Check sheet for the modelled part. Datum: model origin and axes. Units: mm. A direction names the side the tool comes from. Coordinates: 2 decimals unless noted, no trailing zeros. Order: outer loops, then holes, each group sorted by start corner. A loop starts at its lowest first (then second) coordinate and runs counter-clockwise, first axis right, second up.
from build123d import *

# Parameters (mm, degrees)
F1_DEPTH = 120
F3_D     = 2.7
F3_DEPTH = 12
F3_TIP   = 0.8111618357
F4_W     = 9
F4_H     = 9
F5_DEPTH = 5
F7_D     = 2.7
F7_DEPTH = 5
F7_TIP   = 0.8111618357
F9_DEPTH = 50


with BuildPart() as f1:
    # F0 (on Front) → F1 (new body)
    with BuildSketch(Plane.XZ):
        with BuildLine():
            Line((-10.0352883258, -17.0069661875), (0, -17.0069661875))
            Line((0, -17.0069661875), (10.0352883258, -17.0069661875))
            Line((10.0352883258, -17.0069661875), (7, -12.5069661875))
            Line((7, -12.5069661875), (46.25, -12.5069661875))
            Line((46.25, -12.5069661875), (43.2147116742, -17.0069661875))
            Line((43.2147116742, -17.0069661875), (53.2852883258, -17.0069661875))
            Line((53.2852883258, -17.0069661875), (50.25, -12.5069661875))
            Line((50.25, -12.5069661875), (55.25, -12.5069661875))
            ThreePointArc((55.25, -12.5069661875), (57.3713203436, -11.6282865311), (58.25, -9.5069661875))
            Line((58.25, -9.5069661875), (58.25, 21.9930338125))
            ThreePointArc((58.25, 21.9930338125), (57.3713203436, 24.114354156), (55.25, 24.9930338125))
            Line((55.25, 24.9930338125), (50.8726710718, 24.9930338125))
            Line((50.8726710718, 24.9930338125), (53.5, 20.9930338125))
            Line((53.5, 20.9930338125), (48.25, 20.9930338125))
            Line((48.25, 20.9930338125), (48.25, 1.6930338125))
            Line((48.25, 1.6930338125), (51.1, 1.6930338125))
            Line((51.1, 1.6930338125), (51.1, -0.5069661875))
            Line((51.1, -0.5069661875), (48.25, -0.5069661875))
            Line((48.25, -0.5069661875), (48.25, -3.5069661875))
            ThreePointArc((48.25, -3.5069661875), (47.3713203436, -5.6282865311), (45.25, -6.5069661875))
            Line((45.25, -6.5069661875), (0, -6.5069661875))
            Line((0, -6.5069661875), (-45.25, -6.5069661875))
            ThreePointArc((-45.25, -6.5069661875), (-47.3713203436, -5.6282865311), (-48.25, -3.5069661875))
            Line((-48.25, -3.5069661875), (-48.25, -0.5069661875))
            Line((-48.25, -0.5069661875), (-51.1, -0.5069661875))
            Line((-51.1, -0.5069661875), (-51.1, 1.6930338125))
            Line((-51.1, 1.6930338125), (-48.25, 1.6930338125))
            Line((-48.25, 1.6930338125), (-48.25, 20.9930338125))
            Line((-48.25, 20.9930338125), (-53.5, 20.9930338125))
            Line((-53.5, 20.9930338125), (-50.8726710718, 24.9930338125))
            Line((-50.8726710718, 24.9930338125), (-55.25, 24.9930338125))
            ThreePointArc((-55.25, 24.9930338125), (-57.3713203436, 24.114354156), (-58.25, 21.9930338125))
            Line((-58.25, 21.9930338125), (-58.25, -9.5069661875))
            ThreePointArc((-58.25, -9.5069661875), (-57.3713203436, -11.6282865311), (-55.25, -12.5069661875))
            Line((-55.25, -12.5069661875), (-50.25, -12.5069661875))
            Line((-50.25, -12.5069661875), (-53.2852883258, -17.0069661875))
            Line((-53.2852883258, -17.0069661875), (-43.2147116742, -17.0069661875))
            Line((-43.2147116742, -17.0069661875), (-46.25, -12.5069661875))
            Line((-46.25, -12.5069661875), (-7, -12.5069661875))
            Line((-7, -12.5069661875), (-10.0352883258, -17.0069661875))
        make_face()
        Polygon((-54, -3.1069661875), (-54, -1.4069661875), (-52.4, -1.4069661875), (-52.4, -3.1069661875), (-50.7, -3.1069661875), (-50.7, -4.7069661875), (-52.4, -4.7069661875), (-52.4, -6.4069661875), (-54, -6.4069661875), (-54, -4.7069661875), (-55.7, -4.7069661875), (-55.7, -3.1069661875), align=None, mode=Mode.SUBTRACT)
        Polygon((52.4, -1.4069661875), (54, -1.4069661875), (54, -3.1069661875), (55.7, -3.1069661875), (55.7, -4.7069661875), (54, -4.7069661875), (54, -6.4069661875), (52.4, -6.4069661875), (52.4, -4.7069661875), (50.7, -4.7069661875), (50.7, -3.1069661875), (52.4, -3.1069661875), align=None, mode=Mode.SUBTRACT)
        Polygon((-55.7, 15.5930338125), (-55.7, 17.1930338125), (-54, 17.1930338125), (-54, 18.8930338125), (-52.4, 18.8930338125), (-52.4, 17.1930338125), (-50.7, 17.1930338125), (-50.7, 15.5930338125), (-52.4, 15.5930338125), (-52.4, 13.8930338125), (-54, 13.8930338125), (-54, 15.5930338125), align=None, mode=Mode.SUBTRACT)
        Polygon((54, 18.8930338125), (54, 17.1930338125), (55.7, 17.1930338125), (55.7, 15.5930338125), (54, 15.5930338125), (54, 13.8930338125), (52.4, 13.8930338125), (52.4, 15.5930338125), (50.7, 15.5930338125), (50.7, 17.1930338125), (52.4, 17.1930338125), (52.4, 18.8930338125), align=None, mode=Mode.SUBTRACT)
    extrude(amount=-F1_DEPTH)

    # F3
    with Locations(Plane.XZ):
        with Locations((0, -15.5069661875)):
            Hole(F3_D / 2, depth=F3_DEPTH)
            with Locations((0, 0, -(F3_DEPTH + F3_TIP / 2))):  # 118° drill point
                Cone(0, F3_D / 2, F3_TIP, mode=Mode.SUBTRACT)

    # F4 (on face) → F5 (join)
    with BuildSketch(Plane.XY.offset(-6.5069661875)):
        with Locations((-10.75, 14.5)):
            Rectangle(F4_W, F4_H)
        with Locations((-10.75, 106.5)):
            Rectangle(F4_W, F4_H)
        with Locations((37.25, 14.5)):
            Rectangle(F4_W, F4_H)
        with Locations((37.25, 106.5)):
            Rectangle(F4_W, F4_H)
    extrude(amount=F5_DEPTH)

    # F7
    with Locations(Plane.XY.offset(-1.5069661875)):
        with Locations((-10.75, 106.5), (37.25, 106.5), (-10.75, 14.5), (37.25, 14.5)):
            Hole(F7_D / 2, depth=F7_DEPTH)
            with Locations((0, 0, -(F7_DEPTH + F7_TIP / 2))):  # 118° drill point
                Cone(0, F7_D / 2, F7_TIP, mode=Mode.SUBTRACT)

    # F8 (on face) → F9 (join)
    with BuildSketch(Plane(origin=(0, 120, 0), x_dir=(-1, 0, 0), z_dir=(0, 1, 0))):
        Polygon((21.25, -1.0069661875), (21.25, -6.5069661875), (25.5, -6.5069661875), (25.5, -4.5069661875), (22.75, -4.5069661875), (22.75, -2.7069661875), (25.5, -2.7069661875), (25.5, -1.0069661875), align=None)
        Polygon((41, -4.5069661875), (41, -6.5069661875), (45.25, -6.5069661875), (45.25, -1.0069661875), (41, -1.0069661875), (41, -2.7069661875), (43.75, -2.7069661875), (43.75, -4.5069661875), align=None)
    extrude(amount=-F9_DEPTH)


solid = f1.part
(1) Release check for a two-part mould opening along Y. For faces 1 (the conical face through (37.47, 14.57, -7.18)), 2 (the cylindrical face through (0.18, 6.08, -14.17)), 3 (the cylindrical face through (-11.37, 105.3, -4.04)) record: +Y half, -Y half, draft (parallel to the pull), parting line (faces both ways), or undercut.
Filled in:
face 1: undercut
face 2: draft
face 3: undercut
(2) Cross-section at A-A (z = 11.5). Enter the section's corners in (x, y).
Filled in:
outline: (-58.25, 0) - (-48.25, 0) - (-48.25, 120) - (-58.25, 120) - close; (48.25, 0) - (58.25, 0) - (58.25, 120) - (48.25, 120) - close
(3) Cross-section at B-B (y = 49). Count the separate pieces of the cut face and the enclosed holes in it, and give its area (3 significant figures).
Filled in:
separate pieces: 1
enclosed holes: 4
area: 1,370 mm2
(4) Cross-section at C-C (x = -4). Enter the section's corners in (y, z).
Filled in:
outline: (0, -17.01) - (120, -17.01) - (120, -6.51) - (0, -6.51) - close
(5) Go/stop test with flat-tipped pins: P1, Ø0.9, axis at x = 54.5, y = 31, coming from the -Z side; P2, Ø10, axis at x = -11.5, y = 107, coming from the +Z side; P3, Ø2, axis at x = -4.5, y = 47.5, coming from the +Z side. Record where each tip stops, or that it passes through.
Filled in:
P1: stops at z = -12.51
P2: stops at z = -1.51
P3: stops at z = -6.51
(6) Tool access check on faces 4 (the flat face through (-11, 19, -4)), 5 (the flat face through (-12, 108, -1.507)), 6 (the flat face through (-48, 59, -17.007)), 7 (the flat face through (58.25, 59, 6)). Record the directions out of +Z, -Z, +X, -X, +Y, -Y that give a thin tool (end or side, any length) a straight path to the whole face; none if there is none.
Filled in:
face 4: +Z
face 5: +Z, +Y, -Y
face 6: -Z, +X, -X, +Y, -Y
face 7: +Z, -Z, +X, +Y, -Y
(7) Thickness scan on probe 1 along X at (y, z) = (25, -3.5); probe 2 along Y at (x, z) = (-10, -5); probe 3 along X at (y, z) = (85.5, 7.5). Record the ranges inside material, lowest first.
Filled in:
probe 1: x = -58.25 to -55.7, -50.7 to -48.25, 48.25 to 50.7, 55.7 to 58.25
probe 2: y = 10 to 13.38, 15.62 to 19, 102 to 105.38, 107.62 to 111
probe 3: x = -58.25 to -48.25, 48.25 to 58.25
